Design review of the part built by this model. Coordinates are the model's own, in mm. Face numbers are marked on the shaded views. A direction names the side the tool comes from. Coordinates: 2 decimals unless noted, no trailing zeros. Write each loop counter-clockwise with the first axis right and the second up, starting at its lowest first coordinate (ties: lowest second). Pieces come first, ordered by that corner, then holes. Notation, with made-up numbers: (38.25, 74.25) - (60.25, 74.25) arc R26 ccw to (60.25, 105.25) - close; hole circle Ø2 at (75.25, 38.5). An arc over 180 degrees is marked (long way). Answer as a JSON object with one key per item and string values.
```python
from build123d import *

# Parameters (mm, degrees)
SKETCH1_R              = 25
BOSS_EXTRUDE1_DEPTH    = 50
SKETCH2_R              = 25
SKETCH2_R_2            = 18
CUT_EXTRUDE1_DEPTH     = 46
CUT_EXTRUDE2_START     = -4
CUT_EXTRUDE2_OUTLINE_R = 1.5
CUT_EXTRUDE2_DEPTH     = 4
SKETCH6_R              = 6.5
CUT_EXTRUDE5_DEPTH     = 5
SKETCH8_R              = 11
CUT_EXTRUDE6_DEPTH     = 13
SKETCH9_R              = 11
CUT_EXTRUDE7_DEPTH     = 5
SKETCH10_R             = 4
CUT_EXTRUDE8_DEPTH     = 58.37612744
SKETCH11_R             = 11
SKETCH11_R_2           = 4
CUT_EXTRUDE9_DEPTH     = 27
SKETCH13_R             = 18
SKETCH13_R_2           = 11
CUT_EXTRUDE10_DEPTH    = 18
CUT_EXTRUDE13_START    = -3
CUT_EXTRUDE13_DEPTH    = 3
BOSS_EXTRUDE4_START    = 2
SKETCH19_R             = 1.5
SKETCH19_R_2           = 18
BOSS_EXTRUDE4_DEPTH    = 2
F_3DSKETCH11_R         = 1.5
CUT_EXTRUDE14_DEPTH    = 19.9
SKETCH20_R             = 11
CUT_EXTRUDE15_DEPTH    = 5
SKETCH21_R             = 17
BOSS_EXTRUDE5_DEPTH    = 1.5


with BuildPart() as part:
    # Sketch1 → Boss-Extrude1 (new body)
    with BuildSketch(Plane(origin=(0, 0, 0), x_dir=(1, 0, 0), z_dir=(0, 1, 0))):
        with Locations(Location((0, 0, 0), (0, 0, 270))):
            Circle(SKETCH1_R)
    extrude(amount=BOSS_EXTRUDE1_DEPTH)

    # Sketch2 → Cut-Extrude1 (cut)
    with BuildSketch(Plane.XZ):
        with Locations(Location((0, 0, 0), (0, 0, 90))):
            Circle(SKETCH2_R)
        with Locations(Location((0, 0, 0), (0, 0, 270))):
            Circle(SKETCH2_R_2, mode=Mode.SUBTRACT)
    extrude(amount=-CUT_EXTRUDE1_DEPTH, mode=Mode.SUBTRACT)

    # Cut-Extrude2: read off the stored shape, not the designer's step
    # Cut-Extrude2 outline → Cut-Extrude2 (cut)
    with BuildSketch(Plane(origin=(0, 50, 0), x_dir=(1, 0, 0), z_dir=(0, 1, 0)).offset(CUT_EXTRUDE2_START)):
        with BuildLine():
            ThreePointArc((-15.132415538, -19.9), (0, -25), (15.132415538, -19.9))
            Line((15.132415538, -19.9), (-15.132415538, -19.9))
        make_face()
        with BuildLine():
            Line((19.9, 15.132415538), (19.9, -15.132415538))
            ThreePointArc((19.9, -15.132415538), (25, 0), (19.9, 15.132415538))
        make_face()
        with BuildLine():
            ThreePointArc((-19.9, 15.132415538), (-25, 0), (-19.9, -15.132415538))
            Line((-19.9, -15.132415538), (-19.9, 15.132415538))
        make_face()
        with BuildLine():
            Line((-15.132415538, 19.9), (15.132415538, 19.9))
            ThreePointArc((15.132415538, 19.9), (0, 25), (-15.132415538, 19.9))
        make_face()
        with Locations((-15.132415538, -15.132415538)):
            Circle(CUT_EXTRUDE2_OUTLINE_R)
        with Locations((15.132415538, -15.132415538)):
            Circle(CUT_EXTRUDE2_OUTLINE_R)
        with Locations((-15.132415538, 15.132415538)):
            Circle(CUT_EXTRUDE2_OUTLINE_R)
        with Locations((15.132415538, 15.132415538)):
            Circle(CUT_EXTRUDE2_OUTLINE_R)
    extrude(amount=CUT_EXTRUDE2_DEPTH, mode=Mode.SUBTRACT)

    # Sketch6 → Cut-Extrude5 (cut)
    with BuildSketch(Plane(origin=(0, 50, 0), x_dir=(1, 0, 0), z_dir=(0, 1, 0))):
        with Locations(Location((0, 0, 0), (0, 0, 270))):
            Circle(SKETCH6_R)
    extrude(amount=-CUT_EXTRUDE5_DEPTH, mode=Mode.SUBTRACT)

    # Sketch8 → Cut-Extrude6 (cut)
    with BuildSketch(Plane(origin=(0, 45, 0), x_dir=(1, 0, 0), z_dir=(0, 1, 0))):
        with Locations(Location((0, 0, 0), (0, 0, 270))):
            Circle(SKETCH8_R)
    extrude(amount=-CUT_EXTRUDE6_DEPTH, mode=Mode.SUBTRACT)

    # Sketch9 → Cut-Extrude7 (cut)
    with BuildSketch(Plane(origin=(0, 50, 0), x_dir=(1, 0, 0), z_dir=(0, 1, 0))):
        with Locations(Location((0, 0, 0), (0, 0, 270))):
            Circle(SKETCH9_R)
    extrude(amount=-CUT_EXTRUDE7_DEPTH, mode=Mode.SUBTRACT)

    # Sketch10 → Cut-Extrude8 (cut, through all)
    with BuildSketch(Plane.XZ):
        with Locations(Location((0, 0, 0), (0, 0, 270))):
            Circle(SKETCH10_R)
    extrude(amount=-CUT_EXTRUDE8_DEPTH, mode=Mode.SUBTRACT)

    # Sketch11 → Cut-Extrude9 (cut)
    with BuildSketch(Plane.XZ):
        with Locations(Location((0, 0, 0), (0, 0, 90))):
            Circle(SKETCH11_R)
        with Locations(Location((0, 0, 0), (0, 0, 270))):
            Circle(SKETCH11_R_2, mode=Mode.SUBTRACT)
    extrude(amount=-CUT_EXTRUDE9_DEPTH, mode=Mode.SUBTRACT)

    # Sketch13 → Cut-Extrude10 (cut)
    with BuildSketch(Plane.XZ):
        with Locations(Location((0, 0, 0), (0, 0, 270))):
            Circle(SKETCH13_R)
        with Locations(Location((0, 0, 0), (0, 0, 270))):
            Circle(SKETCH13_R_2, mode=Mode.SUBTRACT)
    extrude(amount=-CUT_EXTRUDE10_DEPTH, mode=Mode.SUBTRACT)

    # Sketch18 → Cut-Extrude13 (cut)
    with BuildSketch(Plane(origin=(0, 50, 0), x_dir=(1, 0, 0), z_dir=(0, 1, 0)).offset(CUT_EXTRUDE13_START)):
        with BuildLine():
            Line((-19.9, 15.132415538), (-19.9, -15.132415538))
            ThreePointArc((-19.9, -15.132415538), (-17.67766953, -17.67766953), (-15.132415538, -19.9))
            Line((-15.132415538, -19.9), (15.132415538, -19.9))
            ThreePointArc((15.132415538, -19.9), (17.67766953, -17.67766953), (19.9, -15.132415538))
            Line((19.9, -15.132415538), (19.9, 15.132415538))
            ThreePointArc((19.9, 15.132415538), (17.67766953, 17.67766953), (15.132415538, 19.9))
            Line((15.132415538, 19.9), (-15.132415538, 19.9))
            ThreePointArc((-15.132415538, 19.9), (-17.67766953, 17.67766953), (-19.9, 15.132415538))
        make_face()
    extrude(amount=CUT_EXTRUDE13_DEPTH, mode=Mode.SUBTRACT)

    # Sketch19 → Boss-Extrude4 (add)
    with BuildSketch(Plane.XZ.offset(-46).offset(BOSS_EXTRUDE4_START)):
        with BuildLine():
            ThreePointArc((-15.132415538, 19.9), (-17.67766953, 17.67766953), (-19.9, 15.132415538))
            Line((-19.9, 15.132415538), (-19.9, -15.132415538))
            ThreePointArc((-19.9, -15.132415538), (-17.67766953, -17.67766953), (-15.132415538, -19.9))
            Line((-15.132415538, -19.9), (15.132415538, -19.9))
            ThreePointArc((15.132415538, -19.9), (17.67766953, -17.67766953), (19.9, -15.132415538))
            Line((19.9, -15.132415538), (19.9, 15.132415538))
            ThreePointArc((19.9, 15.132415538), (17.67766953, 17.67766953), (15.132415538, 19.9))
            Line((15.132415538, 19.9), (-15.132415538, 19.9))
        make_face()
        with Locations(Location((-15.132415538, -15.132415538, 0), (0, 0, 90))):
            Circle(SKETCH19_R, mode=Mode.SUBTRACT)
        with Locations(Location((-15.132415538, 15.132415538, 0), (0, 0, 90))):
            Circle(SKETCH19_R, mode=Mode.SUBTRACT)
        with Locations(Location((0, 0, 0), (0, 0, 270))):
            Circle(SKETCH19_R_2, mode=Mode.SUBTRACT)
        with Locations(Location((15.132415538, 15.132415538, 0), (0, 0, 90))):
            Circle(SKETCH19_R, mode=Mode.SUBTRACT)
        with Locations(Location((15.132415538, -15.132415538, 0), (0, 0, 90))):
            Circle(SKETCH19_R, mode=Mode.SUBTRACT)
    extrude(amount=-BOSS_EXTRUDE4_DEPTH)

    # 3DSketch11 → Cut-Extrude14 (cut)
    with BuildSketch(Plane(origin=(0, 44, 0), x_dir=(0, -1, 0), z_dir=(-1, 0, 0))):
        with Locations(Location((2.5, 0, 0), (0, 0, 90))):
            Circle(F_3DSKETCH11_R)
    extrude(amount=CUT_EXTRUDE14_DEPTH, mode=Mode.SUBTRACT)

    # Sketch20 → Cut-Extrude15 (cut)
    with BuildSketch(Plane.XZ.offset(-27)):
        with Locations(Location((0, 0, 0), (0, 0, 270))):
            Circle(SKETCH20_R)
    extrude(amount=-CUT_EXTRUDE15_DEPTH, mode=Mode.SUBTRACT)

    # Sketch21 → Boss-Extrude5 (add)
    with BuildSketch(Plane(origin=(0, 47, 0), x_dir=(1, 0, 0), z_dir=(0, 1, 0))):
        with BuildLine():
            Line((-19.9, 15.132415538), (-19.9, -15.132415538))
            ThreePointArc((-19.9, -15.132415538), (-17.67766953, -17.67766953), (-15.132415538, -19.9))
            Line((-15.132415538, -19.9), (15.132415538, -19.9))
            ThreePointArc((15.132415538, -19.9), (17.67766953, -17.67766953), (19.9, -15.132415538))
            Line((19.9, -15.132415538), (19.9, 15.132415538))
            ThreePointArc((19.9, 15.132415538), (17.67766953, 17.67766953), (15.132415538, 19.9))
            Line((15.132415538, 19.9), (-15.132415538, 19.9))
            ThreePointArc((-15.132415538, 19.9), (-17.67766953, 17.67766953), (-19.9, 15.132415538))
        make_face()
        with Locations(Location((0, 0, 0), (0, 0, 270))):
            Circle(SKETCH21_R, mode=Mode.SUBTRACT)
    extrude(amount=BOSS_EXTRUDE5_DEPTH)


solid = part.part
```
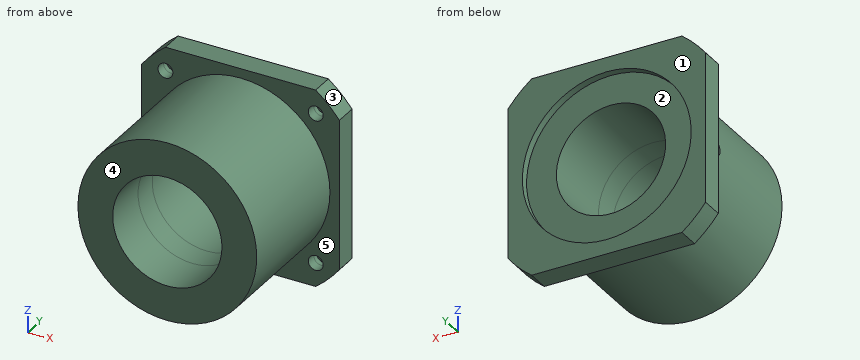
(1) Take a section at C-C, the plane z = 6. Write out the cut boundary in (x, y).
Solved:
{"outline": "(-19.9, 44) - (-16.97, 44) - (-16.97, 18) - (-9.22, 18) - (-9.22, 47) - (-15.91, 47) - (-15.91, 48.5) - (-19.9, 48.5) - close; (9.22, 18) - (16.97, 18) - (16.97, 44) - (19.9, 44) - (19.9, 48.5) - (15.91, 48.5) - (15.91, 47) - (9.22, 47) - close"}
(2) Take a section at B-B, the plane x = 6.5. Write out the cut boundary in (y, z), and give its area (3 significant figures).
Solved:
{"outline": "(18, -16.79) - (44, -16.79) - (44, -19.9) - (48.5, -19.9) - (48.5, -15.71) - (47, -15.71) - (47, -8.87) - (18, -8.87) - close; (18, 8.87) - (47, 8.87) - (47, 15.71) - (48.5, 15.71) - (48.5, 19.9) - (44, 19.9) - (44, 16.79) - (18, 16.79) - close", "area": "490 mm^2"}
(3) Take a section at A-A, the plane z = 0. Write out the cut boundary in (x, y).
Solved:
{"outline": "(-19.9, 44) - (-18, 44) - (-18, 43) - (-11, 43) - (-11, 47) - (-17, 47) - (-17, 48.5) - (-19.9, 48.5) - close; (-18, 18) - (-11, 18) - (-11, 40) - (-18, 40) - close; (11, 18) - (18, 18) - (18, 44) - (19.9, 44) - (19.9, 48.5) - (17, 48.5) - (17, 47) - (11, 47) - close"}
(4) Tool access review of the marked faces 4 and 5: name each direction out of +Z, -Z, +X, -X, +Y, -Y from which nothing blocks a thin tool from reaching the whole face with its end or side.
Solved:
{"face 4": "+Z, -Z, +X, -X, -Y", "face 5": "-Y"}
(5) The part is to be moulded in two halves that separate along Z. For the marked faces 1, 2 and 3, say which applies: pulls with the +Z half, pulls with the -Z half, needs draft (parallel to the pull), parting line crosses it, or undercut.
Solved:
{"face 1": "needs draft", "face 2": "undercut", "face 3": "pulls with the +Z half"}
(6) For pin 1 (2.5 mm diameter, centred on x = 15.13, z = -15.13, fed in from -Y); pin 2 (6 mm diameter, centred on x = 10, z = -11.5, fed in from +Y); pin 3 (8 mm diameter, centred on x = 12.5, y = 39.5, fed in from -Z); pin 4 (5 mm diameter, centred on x = -15.13, z = -15.13, fed in from -Y), all flat-tipped, find the tip position at first contact; note any pin that passes through.
Solved:
{"pin 1": "stops at y = 47", "pin 2": "stops at y = 48.5", "pin 3": "stops at z = -15.87", "pin 4": "stops at y = 44"}
(7) To check wall thickness, follow line 1 (X direction, y = 22, z = 0); line 2 (X direction, y = 45.5, z = 14.5); line 3 (Y direction, x = 10, z = -7.5). State the ranges of each line that lie inside material, in increasing order. Write a range as from..to.
Solved:
{"line 1": "x = -18..-11, 11..18", "line 2": "x = -19.9..-16.49, -13.77..13.77, 16.49..19.9", "line 3": "y = 18..47"}
(8) Take a section at D-D, the plane y = 39. Write out the cut boundary in (x, z), and give its area (3 significant figures).
Solved:
{"outline": "circle Ø36 at (0, 0); hole circle Ø22 at (0, 0)", "area": "638 mm^2"}
